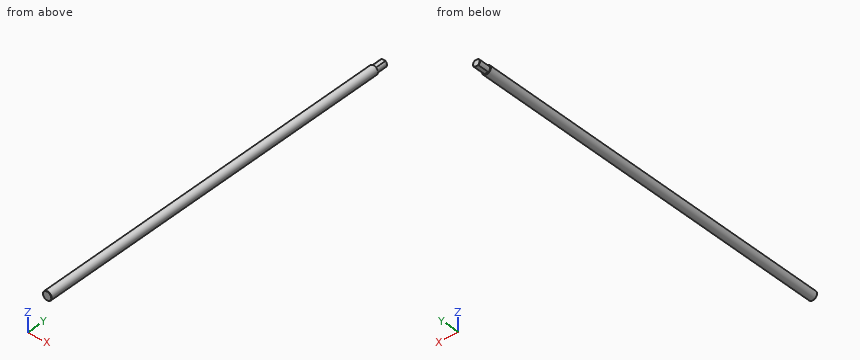
from build123d import *

# Parameters (mm, degrees)
SKETCH1_R               = 7.5
BOSS_EXTRUDE1_DEPTH     = 640
SKETCH2_R               = 6
BOSS_EXTRUDE2_DEPTH     = 20
CHAMFER1_SIZE           = 0.5
CHAMFER2_SIZE           = 0.5
CUT_EXTRUDE1_DEPTH      = 8.5
CUT_EXTRUDE1_DEPTH_BACK = 8.5


with BuildPart() as part:
    # Sketch1 → Boss-Extrude1 (new body)
    with BuildSketch(Plane(origin=(0, 0, 0), x_dir=(1, 0, 0), z_dir=(0, 1, 0))):
        Circle(SKETCH1_R)
    extrude(amount=BOSS_EXTRUDE1_DEPTH)

    # Sketch2 → Boss-Extrude2 (add)
    with BuildSketch(Plane(origin=(0, 640, 0), x_dir=(1, 0, 0), z_dir=(0, 1, 0))):
        Circle(SKETCH2_R)
    extrude(amount=BOSS_EXTRUDE2_DEPTH)

    # Chamfer1
    chamfer1_edges = [part.edges().sort_by_distance(p)[0] for p in [
        (-6, 660, 0),
    ]]
    chamfer(chamfer1_edges, length=CHAMFER1_SIZE)

    # Chamfer2
    chamfer2_edges = [part.edges().sort_by_distance(p)[0] for p in [
        (-7.5, 0, 0),
    ]]
    chamfer(chamfer2_edges, length=CHAMFER2_SIZE)

    # Sketch3 → Cut-Extrude1 (cut, two sides)
    with BuildSketch(Plane(origin=(0, 0, 0), x_dir=(0, 0, -1), z_dir=(1, 0, 0))) as cut_extrude1_sk:
        Polygon((11.720103358, 640), (5, 640), (5, 665.518180004), (13.892257978, 665.518180004), (13.892257978, 640), align=None)
        Polygon((-13.892257978, 640), (-11.720103358, 640), (-5, 640), (-5, 665.518180004), (-13.892257978, 665.518180004), align=None)
    extrude(amount=CUT_EXTRUDE1_DEPTH, mode=Mode.SUBTRACT)
    extrude(cut_extrude1_sk.sketch, amount=-CUT_EXTRUDE1_DEPTH_BACK, mode=Mode.SUBTRACT)


solid = part.part
Input: part model. Units: mm. Frame: model coordinates. Give positions to 0.01 mm unless a question says otherwise; leave off trailing zeros. Loops run counter-clockwise (first coordinate to the right, second up) from the corner with the lowest first, then second, coordinate; pieces in that order, holes last. Notation, with made-up numbers: M -18,-9.5 L -10,-9.5 A12 cw -10,13.5 Z; hole C 74.25,-6.75 d4. An arc over 180 degrees is marked long. Use CSV: the item, a comma, the result in double quotes.
(1) Pin query (flat end, axial travel): P1, Ø1, axis at x = 1.5, y = 238, coming from the +Z side; P2, Ø2, axis at x = -1, y = 647, coming from the +Z side; P3, Ø6, axis at x = 3, z = -4, coming from the -Y side; P4, Ø8, axis at x = 6, y = 591.5, coming from the -Z side. Return the tip coordinate at first contact, or that it passes through.
Outcome:
P1,"stops at z = 7.43"
P2,"stops at z = 5"
P3,"stops at y = 0"
P4,"stops at z = -7.23"
(2) Section A-A, the plane y = 213. Return loops of the section in (x, z), plus the area to 3 significant figures.
Outcome:
outline,"C 0,0 d15"
area,"177 mm²"
(3) Material intervals for L1, parallel to X at y = 184, z = 2.5; L2, parallel to X at y = 81.5, z = 5; L3, parallel to Z at x = 2.75, y = 355, sorted ascending. Write a range as [from, to].
Outcome:
L1,"x = [-7.07, 7.07]"
L2,"x = [-5.59, 5.59]"
L3,"z = [-6.98, 6.98]"
